from build123d import *

# Parameters (mm, degrees)
BOSS_EXTRUDE1_DEPTH = 12.7
SKETCH2_R           = 2.54
CUT_EXTRUDE1_DEPTH  = 3.175


with BuildPart() as part:
    # Sketch1 → Boss-Extrude1 (new body)
    with BuildSketch(Plane(origin=(0, 0, 0), x_dir=(0, 0, -1), z_dir=(1, 0, 0))):
        Polygon((1.27, 3.81), (0, 16.51), (-1.27, 3.81), (-5.08, 3.81), (-5.08, 0), (5.08, 0), (5.08, 3.81), align=None)
    extrude(amount=BOSS_EXTRUDE1_DEPTH)

    # Sketch2 → Cut-Extrude1 (cut)
    with BuildSketch(Plane.XZ):
        with Locations((6.35, 0)):
            Circle(SKETCH2_R)
    extrude(amount=-CUT_EXTRUDE1_DEPTH, mode=Mode.SUBTRACT)


solid = part.part
Geometry: final body of the model. Coordinates: model frame, mm. A direction names the side the tool comes from. Give positions to 0.01 mm unless a question says otherwise; leave off trailing zeros. Write each loop counter-clockwise with the first axis right and the second up, starting at its lowest first coordinate (ties: lowest second). Pieces come first, ordered by that corner, then holes. Notation, with made-up numbers: (25, 69) - (60, 69) arc R17 cw to (60, 84) - close; hole circle Ø5 at (88, 40). An arc over 180 degrees is marked (long way). Return JSON: item names as keys, results as strings. Group by question number.
1) Section D-D on x = 3. Return the cut outline in (y, z).
2) Set-up query: faces 4 (the cylindrical face through (4.48, 1.57, 1.72)), 5 (the flat face through (6, 2, -5.08)), 6 (the flat face through (6, 3.81, 3)), 7 (the flat face through (6, 3.81, -3)). Return all of +Z, -Z, +X, -X, +Y, -Y with unobstructed straight access to the full face (end or side cutting, diameter ignored); none if empty.
3) Line query: line 1 (Z direction, x = 6.35, y = 0.8); line 2 (Y direction, x = 12.25, z = -1.5); line 3 (Y direction, x = 4.75, z = 1.75) (3 decimals). Output: solid intervals per line, ascending.
4) Section B-B on y = 1.5. Return the cut outline in (x, z).
5) Section A-A on x = 6.35. Return the cut outline in (y, z) (3 decimals).
6) Section C-C on z = 0.25. Return the cut outline in (x, y) (3 decimals), plus the area to 3 significant figures.
7) Mould query, pull axis X, two halves, no side actions, for faces 1 (the flat face through (6, 2, 5.08)), 2 (the flat face through (0, 3, 0)), 3 (the flat face through (6, 3.175, 0)). Classes: released by +X, released by -X, zero draft, split by the parting line, or undercut.
8) First-contact query: P1, Ø6, axis at x = 6.5, y = 14, coming from the +Z side; P2, Ø1.5, axis at x = 5.5, z = 0.5, coming from the -Y side (3 decimals); P3, Ø1.1, axis at x = 8, z = -4, coming from the +Y side; P4, Ø1.5, axis at y = 15, z = -1, coming from the -X side. Flat tips, straight axial feed; report the tip coordinate or a pass-through.
Filled in:
{
 "1": {"outline": "(0, -5.08) - (3.81, -5.08) - (3.81, -1.27) - (16.51, 0) - (3.81, 1.27) - (3.81, 5.08) - (0, 5.08) - close"},
 "2": {"face 4": "-Y", "face 5": "-Z, +X, -X, +Y, -Y", "face 6": "+Z, +X, -X, +Y", "face 7": "-Z, +X, -X, +Y"},
 "3": {"line 1": "z = -5.08 to -2.54, 2.54 to 5.08", "line 2": "y = 0 to 3.81", "line 3": "y = 3.175 to 3.81"},
 "4": {"outline": "(0, -5.08) - (12.7, -5.08) - (12.7, 5.08) - (0, 5.08) - close; hole circle Ø5.08 at (6.35, 0)"},
 "5": {"outline": "(0, -5.08) - (3.81, -5.08) - (3.81, -1.27) - (16.51, 0) - (3.81, 1.27) - (3.81, 5.08) - (0, 5.08) - (0, 2.54) - (3.175, 2.54) - (3.175, -2.54) - (0, -2.54) - close"},
 "6": {"outline": "(0, 0) - (3.822, 0) - (3.822, 3.175) - (8.878, 3.175) - (8.878, 0) - (12.7, 0) - (12.7, 14.01) - (0, 14.01) - close", "area": "162 mm^2"},
 "7": {"face 1": "zero draft", "face 2": "released by -X", "face 3": "undercut"},
 "8": {"P1": "stops at z = 0.55", "P2": "stops at y = 3.175", "P3": "stops at y = 3.81", "P4": "passes through"}
}
